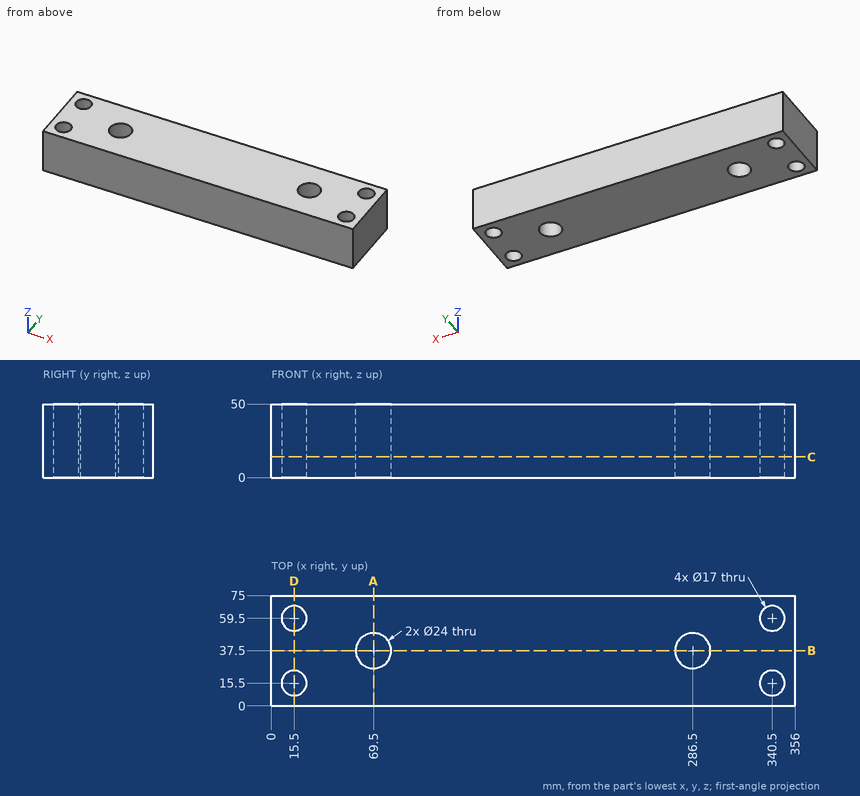
Answer from the drawing. Dimensions are ordinates in mm from the lowest x, y and z of the part. Round coordinates to 2 decimals unless told otherwise and drop trailing zeros. Order: outer loops, then holes, each group sorted by start corner. A loop starts at its lowest first (then second) coordinate and runs counter-clockwise, first axis right, second up.
1) The part is cut by section A-A on x = 69.5. Write down the section's boundary in (y, z).
2) The part is cut by section D-D on x = 15.5. Write down the section's boundary in (y, z).
3) The part is cut by section C-C on z = 14. Write down the section's boundary in (x, y), plus the area to 3 significant figures.
4) The part is cut by section B-B on y = 37.5. Write down the section's boundary in (x, z).
5) Straight lines are drawn through the part: L1, parallel to X at y = 37.5, z = 21; L2, parallel to X at y = 59, z = 23; L3, parallel to Y at x = 340.5, z = 12. For each, find the intervals that lie inside material, in ascending order.
Resolved:
1. outline: (0, 0) - (25.5, 0) - (25.5, 50) - (0, 50) - close; (49.5, 0) - (75, 0) - (75, 50) - (49.5, 50) - close
2. outline: (0, 0) - (7, 0) - (7, 50) - (0, 50) - close; (24, 0) - (51, 0) - (51, 50) - (24, 50) - close; (68, 0) - (75, 0) - (75, 50) - (68, 50) - close
3. outline: (0, 0) - (356, 0) - (356, 75) - (0, 75) - close; hole circle Ø17 at (15.5, 15.5); hole circle Ø17 at (15.5, 59.5); hole circle Ø24 at (69.5, 37.5); hole circle Ø24 at (286.5, 37.5); hole circle Ø17 at (340.5, 15.5); hole circle Ø17 at (340.5, 59.5)
3. area: 24,900 mm2
4. outline: (0, 0) - (57.5, 0) - (57.5, 50) - (0, 50) - close; (81.5, 0) - (274.5, 0) - (274.5, 50) - (81.5, 50) - close; (298.5, 0) - (356, 0) - (356, 50) - (298.5, 50) - close
5. L1: x = 0 to 57.5, 81.5 to 274.5, 298.5 to 356
5. L2: x = 0 to 7.01, 23.99 to 332.01, 348.99 to 356
5. L3: y = 0 to 7, 24 to 51, 68 to 75
